Check sheet for the modelled part. Datum: model origin and axes. Units: mm. A direction names the side the tool comes from. Coordinates: 2 decimals unless noted, no trailing zeros. Loops run counter-clockwise (first coordinate to the right, second up) from the corner with the lowest first, then second, coordinate; pieces in that order, holes last. Notation, with made-up numbers: (-29, 85) - (21, 85) arc R28 ccw to (21, 110) - close; hole circle Ø9 at (66, -23). An arc over 180 degrees is marked (long way). Use a Markdown table: item, result. Add a question column.
1) Draft check along Z on faces 6 (the cylindrical face through (42.25, 8.33, -1.31)), 7 (the flat face through (-2, 16, 1)), 8 (the flat face through (44, 2, 3.5)), 9 (the cylindrical face through (-1, 7, -5)). Enter one of: pulls with the +Z half, pulls with the -Z half, needs draft (parallel to the pull), parting line crosses it, or undercut.
2) Thickness scan on line 1 (X direction, y = 5, z = 0); line 2 (Z direction, x = 18, y = 6); line 3 (Z direction, x = 16, y = 53.5). Record the ranges inside material, lowest first.
3) Go/stop test with flat-tipped pins: P1, Ø0.6, axis at x = 32, z = 4.5, coming from the -Y side; P2, Ø1, axis at x = 24, z = 0.5, coming from the -Y side; P3, Ø1.6, axis at x = -0.5, z = -1.5, coming from the +Y side; P4, Ø4, axis at y = 20, z = -3.5, coming from the +X side. Record where each tip stops, or that it passes through.
4) Sectioned sample at D-D, the plane x = 28. Enter the section's corners in (y, z), then the cut area to 3 significant figures.
5) Sectioned sample at A-A, the plane y = 36.5. Enter the section's corners in (x, z).
6) Sectioned sample at B-B, the plane x = 21.25. Enter the section's corners in (y, z), then the cut area to 3 significant figures.
7) Tool access check on faces 1 (the cylindrical face through (21.717, 53.495, 1.726)), 2 (the cylindrical face through (0.25, 8.33, -1.31)), 3 (the flat face through (-1, 2, 3.5)), 4 (the flat face through (-1, 10, -1)), 5 (the flat face through (44, 4, -1)). Record the directions out of +Z, -Z, +X, -X, +Y, -Y that give a thin tool (end or side, any length) a straight path to the whole face; none if there is none.
8) Sectioned sample at C-C, the plane y = 21. Enter the section's corners in (x, z), then the cut area to 3 significant figures.
from build123d import *

# Parameters (mm, degrees)
BOSS_EXTRUDE1_DEPTH  = 3.5
BOSS_EXTRUDE2_DEPTH  = 2
BOSS_EXTRUDE3_DEPTH  = 2
SKETCH4_R            = 1.5
BOSS_EXTRUDE4_DEPTH  = 1.5
FILLET1_R            = 1
FILLET1_OF_MIRROR1_R = 1


with BuildPart() as part:
    # Sketch1 → Boss-Extrude1 (new body)
    with BuildSketch(Plane.XY):
        with BuildLine():
            Line((42.5, 0), (42.5, 32.25))
            ThreePointArc((42.5, 32.25), (21.25, 53.5), (0, 32.25))
            Line((0, 32.25), (0, 0))
            Line((0, 0), (-2, 0))
            Line((-2, 0), (-2, 32.25))
            ThreePointArc((-2, 32.25), (21.25, 55.5), (44.5, 32.25))
            Line((44.5, 32.25), (44.5, 0))
            Line((44.5, 0), (42.5, 0))
        make_face()
    boss_extrude1 = extrude(amount=BOSS_EXTRUDE1_DEPTH)

    # Sketch2 → Boss-Extrude2 (add)
    with BuildSketch(Plane.XY.offset(3.5)):
        with BuildLine():
            Line((-2, 3), (44.5, 3))
            Line((44.5, 3), (44.5, 32.25))
            ThreePointArc((44.5, 32.25), (21.25, 55.5), (-2, 32.25))
            Line((-2, 32.25), (-2, 3))
        make_face()
    extrude(amount=BOSS_EXTRUDE2_DEPTH)

    # Sketch3 → Boss-Extrude3 (add)
    with BuildSketch(Plane.ZY.offset(2)):
        with BuildLine():
            Line((0, 4), (-2, 4))
            ThreePointArc((-2, 4), (-5, 7), (-2, 10))
            Line((-2, 10), (0, 10))
            Line((0, 10), (0, 4))
        make_face()
    boss_extrude3 = extrude(amount=-BOSS_EXTRUDE3_DEPTH)

    # Sketch4 → Boss-Extrude4 (add)
    with BuildSketch(Plane(origin=(0, 0, 0), x_dir=(0, 0, -1), z_dir=(1, 0, 0))):
        with Locations(Location((2, 7, 0), (0, 0, 180))):
            Circle(SKETCH4_R)
    boss_extrude4 = extrude(amount=BOSS_EXTRUDE4_DEPTH)

    # Fillet1
    fillet1_edges = [part.edges().sort_by_distance(p)[0] for p in [
        (1.5, 7, -3.5),
    ]]
    fillet(fillet1_edges, radius=FILLET1_R)

    # Mirror1: Boss-Extrude1, Boss-Extrude3, Boss-Extrude4 across plane
    add(boss_extrude1.mirror(Plane(origin=(21.25, 0, 0), x_dir=(0, 0, 1), z_dir=(1, 0, 0))))
    add(boss_extrude3.mirror(Plane(origin=(21.25, 0, 0), x_dir=(0, 0, 1), z_dir=(1, 0, 0))))
    add(boss_extrude4.mirror(Plane(origin=(21.25, 0, 0), x_dir=(0, 0, 1), z_dir=(1, 0, 0))))

    # Fillet1 of Mirror1
    fillet1_of_mirror1_edges = [part.edges().sort_by_distance(p)[0] for p in [
        (41, 7, -3.5),
    ]]
    fillet(fillet1_of_mirror1_edges, radius=FILLET1_OF_MIRROR1_R)


solid = part.part
Solved:
| question | item | result |
|---|---|---|
| 1 | face 6 | undercut |
| 1 | face 7 | needs draft |
| 1 | face 8 | pulls with the +Z half |
| 1 | face 9 | pulls with the -Z half |
| 2 | line 1 | x = -2 to 0, 42.5 to 44.5 |
| 2 | line 2 | z = 3.5 to 5.5 |
| 2 | line 3 | z = 0 to 5.5 |
| 3 | P1 | stops at y = 3 |
| 3 | P2 | stops at y = 53.25 |
| 3 | P3 | stops at y = 10 |
| 3 | P4 | passes through |
| 4 | outline | (3, 3.5) - (52.4, 3.5) - (52.4, 0) - (54.5, 0) - (54.5, 5.5) - (3, 5.5) - close |
| 4 | area | 110 mm2 |
| 5 | outline | (-1.61, 0) - (0.43, 0) - (0.43, 3.5) - (42.07, 3.5) - (42.07, 0) - (44.11, 0) - (44.11, 5.5) - (-1.61, 5.5) - close |
| 6 | outline | (3, 3.5) - (53.5, 3.5) - (53.5, 0) - (55.5, 0) - (55.5, 5.5) - (3, 5.5) - close |
| 6 | area | 112 mm2 |
| 7 | face 1 | -Z, -Y |
| 7 | face 2 | none |
| 7 | face 3 | +Z, +X, -X, -Y |
| 7 | face 4 | -Z, +X, -X, +Y |
| 7 | face 5 | -Z, +X, -X, -Y |
| 8 | outline | (-2, 0) - (0, 0) - (0, 3.5) - (42.5, 3.5) - (42.5, 0) - (44.5, 0) - (44.5, 5.5) - (-2, 5.5) - close |
| 8 | area | 107 mm2 |
